```python
from build123d import *

# Parameters (mm, degrees)
SKETCH1_R           = 1
SKETCH1_R_2         = 11
BOSS_EXTRUDE1_DEPTH = 5.842
CUT_EXTRUDE1_DEPTH  = 39.094507846


with BuildPart() as part:
    # Sketch1 → Boss-Extrude1 (new body)
    with BuildSketch(Plane.XY):
        Polygon((25.4, -21), (-25.4, -21), (-25.4, -19.15), (-31.242, -19.15), (-31.242, -6.45), (-25.4, -6.45), (-25.4, 6.25), (-31.242, 6.25), (-31.242, 18.95), (-25.4, 18.95), (-25.4, 21), (25.4, 21), (25.4, 18.95), (31.242, 18.95), (31.242, 6.25), (25.4, 6.25), (25.4, -6.45), (31.242, -6.45), (31.242, -19.15), (25.4, -19.15), align=None)
        with Locations((-15.5, 15.4)):
            Circle(SKETCH1_R, mode=Mode.SUBTRACT)
        with Locations((15.5, 15.4)):
            Circle(SKETCH1_R, mode=Mode.SUBTRACT)
        with Locations((-15.5, -15.6)):
            Circle(SKETCH1_R, mode=Mode.SUBTRACT)
        with Locations((15.5, -15.6)):
            Circle(SKETCH1_R, mode=Mode.SUBTRACT)
        Circle(SKETCH1_R_2, mode=Mode.SUBTRACT)
    extrude(amount=BOSS_EXTRUDE1_DEPTH)

    # Sketch2 → Cut-Extrude1 (cut, through all)
    with BuildSketch(Plane.XY.offset(5.842)):
        Polygon((-22.225, 1.6526), (-22.225, 2.948), (-19.05, 2.948), (-19.05, 1.6526), (-18.041999984, 1.6526), (-18.041999984, -1.8526), (-19.05, -1.8526), (-19.05, -3.148), (-22.225, -3.148), (-22.225, -1.8526), (-25.4, -1.8526), (-25.4, 1.6526), align=None)
        Polygon((18.041999984, 1.6526), (19.05, 1.6526), (19.05, 2.948), (22.225, 2.948), (22.225, 1.6526), (25.4, 1.6526), (25.4, -1.8526), (22.225, -1.8526), (22.225, -3.148), (19.05, -3.148), (19.05, -1.8526), (18.041999984, -1.8526), align=None)
    extrude(amount=-CUT_EXTRUDE1_DEPTH, mode=Mode.SUBTRACT)


solid = part.part
```
Work out the finished part from the listing and answer in its coordinate system (mm). A direction names the side the tool comes from. Give positions to 0.01 mm unless a question says otherwise; leave off trailing zeros. Loops run counter-clockwise (first coordinate to the right, second up) from the corner with the lowest first, then second, coordinate; pieces in that order, holes last. Notation, with made-up numbers: (71, 81.5) -> (104, 81.5) arc R16 cw to (104, 96.5) -> close; hole circle Ø1 at (65.25, 34). An arc over 180 degrees is marked (long way). Put each result on its own line as item: value. Start each with the question number.
Item 1: The part is cut by section B-B (x = 15.5). Give the vertices of the cut face in (y, z), then the cut area to 3 significant figures.
Item 2: The part is cut by section C-C (y = -9.5). Give the vertices of the cut face in (x, z).
Item 3: The part is cut by section D-D (y = -15.6). Give the vertices of the cut face in (x, z).
Item 4: Each of these flat-tipped pins is pushed along its axis until it touches: P1, Ø1.8, axis at x = 28, z = 2, coming from the -Y side; P2, Ø3, axis at x = 29.5, z = 3.5, coming from the +Y side; P3, Ø1.8, axis at y = 0.5, z = 2, coming from the -X side; P4, Ø2.5, axis at x = -15.5, y = 15.4, coming from the +Z side. Where does it stop, or does it pass through?
Item 5: Find the intervals of material crossed by L1, parallel to Y at x = -15.5, z = 3.9; L2, parallel to Y at x = 27.5, z = 5.3; L3, parallel to Y at x = 0, z = 1.55, in increasing order. Write a range as [from, to].
Item 6: The part is cut by section A-A (x = 0). Give the vertices of the cut face in (y, z), then the cut area to 3 significant figures.
Item 7: The mould has two halves that part along X. Classify faces 1 (the face through (-14.96, -14.76, 2.88)), 2 (the face through (31.242, 13, 3)), 3 (the face through (28, 6.25, 3)): released by +X, released by -X, zero draft, split by the parting line, or undercut.
Item 8: Which of the six approach directions +Z, -Z, +X, -X, +Y, -Y give full straight-line access (tool end or side, diameter ignored) to faces 4 (the face through (-25.4, 20, 3)), 5 (the face through (-19.05, -2.5, 3)), 6 (the face through (-25.4, 4, 3))?
Answers below:
1. outline: (-21, 0) -> (-16.6, 0) -> (-16.6, 5.84) -> (-21, 5.84) -> close; (-14.6, 0) -> (14.4, 0) -> (14.4, 5.84) -> (-14.6, 5.84) -> close; (16.4, 0) -> (21, 0) -> (21, 5.84) -> (16.4, 5.84) -> close
1. area: 222 mm2
2. outline: (-31.24, 0) -> (-5.55, 0) -> (-5.55, 5.84) -> (-31.24, 5.84) -> close; (5.55, 0) -> (31.24, 0) -> (31.24, 5.84) -> (5.55, 5.84) -> close
3. outline: (-31.24, 0) -> (-16.5, 0) -> (-16.5, 5.84) -> (-31.24, 5.84) -> close; (-14.5, 0) -> (14.5, 0) -> (14.5, 5.84) -> (-14.5, 5.84) -> close; (16.5, 0) -> (31.24, 0) -> (31.24, 5.84) -> (16.5, 5.84) -> close
4. P1: y = -19.15
4. P2: y = 18.95
4. P3: x = -18.04
4. P4: z = 5.84
5. L1: [-21, -16.6], [-14.6, 14.4], [16.4, 21]
5. L2: [-19.15, -6.45], [6.25, 18.95]
5. L3: [-21, -11], [11, 21]
6. outline: (-21, 0) -> (-11, 0) -> (-11, 5.84) -> (-21, 5.84) -> close; (11, 0) -> (21, 0) -> (21, 5.84) -> (11, 5.84) -> close
6. area: 117 mm2
7. face 1: undercut
7. face 2: released by +X
7. face 3: zero draft
8. face 4: +Z, -Z, -X, +Y
8. face 5: +Z, -Z
8. face 6: +Z, -Z, -X
